Autodesk Fusion 360 part; units mm, degrees
sketch "Sketch1" plane through (0, 0, 0) normal (0, 0, 1) x (1, 0, 0)
  line L0 (0, 0) -> (28, 0)
  line L1 (28, 0) -> (28, 10)
  line L2 (28, 10) -> (0, 10)
  line L3 (0, 10) -> (0, 0)
  line L4 (2, 0) -> (25.8784, 0)
  line L5 (25.8784, 0) -> (25.8784, 10)
  line L6 (25.8784, 10) -> (2, 10)
  line L7 (2, 10) -> (2, 0)
  line L8 (-5, 0) -> (0, 0)
  line L9 (0, 0) -> (0, 6)
  line L10 (0, 6) -> (-5, 6)
  line L11 (-5, 6) -> (-5, 0)
  line L12 (28, 6) -> (33, 6)
  line L13 (33, 6) -> (33, 0)
  line L14 (33, 0) -> (28, 0)
  line L15 (28, 0) -> (28, 6)
  circle A0 centre (-2.4098, 3) radius 1.2381
  line L16 (13.9392, 10) -> (14, 0) construction
  line L17 (2, 8.5375) -> (25.8784, 8.5375)
  line L18 (25.8784, 8.5375) -> (25.8784, 1.4031)
  line L19 (25.8784, 1.4031) -> (2, 1.4031)
  line L20 (2, 1.4031) -> (2, 8.5375)
  circle A1 centre (30.3721, 3.1993) radius 1.2381
  dimension "d1" = 28
  dimension "d2" = 10
  dimension "d11" = 6
  dimension "d12" = 3
  dimension "d14" = 6
extrude "Extrude1" add sketch "Sketch1" along normal blind 2 contours L3 L8 L9 L10 L11 | L1 L12 L13 L14 L15 makes body 1 at (-2.5008, 0.5884, 0) makes body 2 at (30.4882, 0.6549, 0)
extrude "Extrude2" add sketch "Sketch1" along normal blind 13 contours L0 L2 L3 L7 L9 L20 | L0 L4 L5 L7 L19 | L0 L1 L2 L5 L15 L18 | L2 L5 L6 L7 L17 bodies 1 2
extrude "Extrude3" cut sketch "Sketch1" along normal blind 11 contours L0 L4 L5 L7 L19 | L5 L7 L17 L18 L19 L20 | L2 L5 L6 L7 L17 bodies 1
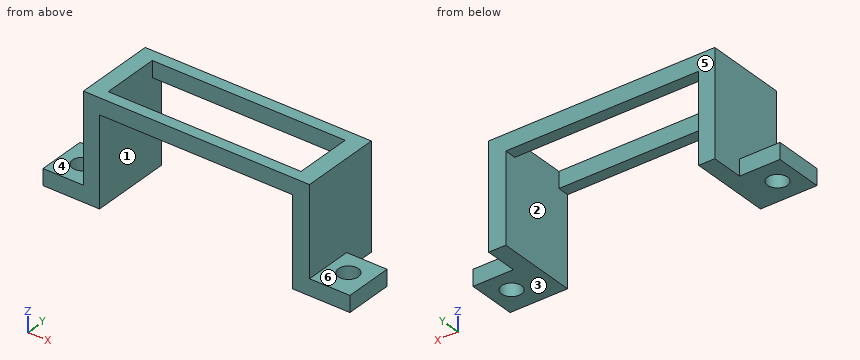
Design review of the part built by this model. Coordinates are the model's own, in mm. Face numbers are marked on the shaded views. A direction names the side the tool comes from. Give positions to 0.01 mm unless a question says otherwise; leave off trailing zeros. Loops run counter-clockwise (first coordinate to the right, second up) from the corner with the lowest first, then second, coordinate; pieces in that order, holes last. Notation, with made-up numbers: M 25.25,-19.75 L 44.25,-19.75 A32 ccw 44.25,10.25 Z; hole C 56.25,-22.75 d11. An arc over 180 degrees is marked long. Answer as a JSON object with one key per item and string values.
Item 1: We need section D-D (z = 11.75). State the section outline as (x, y) points, and give its area (3 significant figures).
Output values:
{"outline": "M 0,0 L 28,0 L 28,10 L 0,10 Z; hole M 2,1.4 L 25.88,1.4 L 25.88,8.54 L 2,8.54 Z", "area": "110 mm2"}
Item 2: Mouldability with a two-part tool opening along X and no side actions: class the marked faces 1, 2 and 3 as pulls with the +X half, pulls with the -X half, needs draft (parallel to the pull), parting line crosses it, or undercut.
Output values:
{"face 1": "undercut", "face 2": "undercut", "face 3": "needs draft"}
Item 3: We need section A-A (z = 4). State the section outline as (x, y) points, and give its area (3 significant figures).
Output values:
{"outline": "M 0,0 L 2,0 L 2,10 L 0,10 Z; M 25.88,0 L 28,0 L 28,10 L 25.88,10 Z", "area": "41.2 mm2"}
Item 4: Wall thickness on line 1 along X through (y, z) = (6, 5.25); line 2 along X through (y, z) = (1.5, 1); line 3 along Y through (x, z) = (18.5, 12.75): over which ranges is each line inside the solid? List them lowest first.
Output values:
{"line 1": "x = 0 to 2, 25.88 to 28", "line 2": "x = -5 to 2, 25.88 to 33", "line 3": "y = 0 to 1.4, 8.54 to 10"}
Item 5: For P1, Ø6, axis at y = 7.5, z = 3, coming from the +X side; P2, Ø1.5, axis at x = 30.37, y = 3.2, coming from the -Z side; P3, Ø1, axis at x = -3.5, z = 0.5, coming from the +Y side; P4, Ø1.5, axis at x = -2, y = 4.5, coming from the +Z side, all flat-tipped, find the tip position at first contact; note any pin that passes through.
Output values:
{"P1": "stops at x = 33", "P2": "passes through", "P3": "stops at y = 6", "P4": "stops at z = 2"}
Item 6: Machinability: for the marked faces 4, 5 and 6, which of the approach directions +Z, -Z, +X, -X, +Y, -Y give a long, thin tool a straight path to every point of the face, cutting with its end or side? Answer none if there is none.
Output values:
{"face 4": "+Z, -X, +Y, -Y", "face 5": "+Z, -Z, +X, -X, +Y", "face 6": "+Z, +X, +Y, -Y"}
Item 7: We need section B-B (x = 16). State the section outline as (y, z) points, and give its area (3 significant figures).
Output values:
{"outline": "M 0,11 L 1.4,11 L 1.4,13 L 0,13 Z; M 8.54,11 L 10,11 L 10,13 L 8.54,13 Z", "area": "5.73 mm2"}
Item 8: We need section C-C (y = 0.5). State the section outline as (x, z) points, and give its area (3 significant figures).
Output values:
{"outline": "M -5,0 L 2,0 L 2,11 L 25.88,11 L 25.88,0 L 33,0 L 33,2 L 28,2 L 28,13 L 0,13 L 0,2 L -5,2 Z", "area": "121 mm2"}
